Here's how the part is built. I have some questions about the finished solid (model axes, mm). A direction names the side the tool comes from. Give positions to 0.01 mm unless a question says otherwise; leave off trailing zeros. Loops run counter-clockwise (first coordinate to the right, second up) from the corner with the lowest first, then second, coordinate; pieces in that order, holes last.
Q1. Suppose I cut it at A-A (x = 51). List the corners of the cut face in (y, z) for me, and give its area (3 significant figures).
Q2. I'm going to push flat-ended pins straight in: P1, Ø19, axis at x = 57, z = -2, coming from the +Y side; P2, Ø8, axis at x = 30.5, y = -11.5, coming from the -Z side; P3, Ø8, axis at y = -11.5, z = -9, coming from the +X side. Where does each tip first touch, or does it pass through?
Q3. Suppose I cut it at C-C (x = 21). List the corners of the cut face in (y, z) for me.
Q4. I need wall thicknesses on probe 1 along Z at (x, y) = (51, -17); probe 2 along Z at (x, y) = (51, 12); probe 3 along Y at (x, z) = (49.5, 15). Which ranges of each line are inside material? Lowest first, please.
Q5. Thinking about a two-plate mould opening in Z: for faces 6 (the face through (20.354, 22.148, 8.24)), 7 (the face through (91, 19.5, 4)), 8 (the face through (48, -9.5, 32)), which applies, pulls with the +Z half, pulls with the -Z half, needs draft (parallel to the pull), parting line crosses it, or undercut?
Q6. Suppose I cut it at D-D (z = 15.5). List the corners of the cut face in (x, y) for me, and give its area (3 significant figures).
Q7. For faces 1 (the face through (18, 19.5, 0)), 2 (the face through (20.354, 22.148, -8.24)), 3 (the face through (23, 23, 0)), 4 (the face through (0, 0, 0)), 5 (the face through (6.2, 24.5, 10.1)), which set-ups out of +Z, -Z, +X, -X, +Y, -Y let a thin tool reach every point of the face, with its end or its side?
Q8. Suppose I cut it at B-B (y = 15). List the corners of the cut face in (x, z) for me.
Autodesk Inventor part; units mm, degrees
ref_plane "Work Plane2" through (0, -9.5, 0) normal (0, 1, 0) x (-1, 0, 0)
ref_plane "YZ Plane" through (0, 0, 0) normal (1, 0, 0) x (0, 1, 0)
ref_plane "XY Plane" through (0, 0, 0) normal (0, 0, 1) x (1, 0, 0)
sketch "Sketch2" plane through (0, 0, 0) normal (1, 0, 0) x (0, 1, 0)
  circle A0 centre (0, 0) radius 26.5
  dimension "d0" = 53
extrude "Extrusion1" add sketch "Sketch2" along normal blind 51
sketch "Sketch3" plane through (0, 0, 0) normal (0, 1, 0) x (-1, 0, 0)
  line L0 (-51, 26.5) -> (-51, -26.5)
  circle A0 centre (-51, 0) radius 48
  circle A1 centre (-51, 0) radius 39
  line L1 (-16.6387, 18.4473) -> (-22.6683, 1.8811)
  circle A2 centre (-17.5, 0) radius 5.5
  line L2 (0, 0) -> (-51, 0) construction
  line L3 (0, 26.5) -> (0, -26.5) construction
  line L4 (-16.6387, -18.4473) -> (-22.6683, -1.8811)
  circle A3 centre (-51, 0) radius 31.5
  point P0 (-22.6683, -1.8811)
  point P1 (-20.4946, 7.8532)
  point P2 (-20.4946, -7.8532)
  dimension "d4" = 78
  dimension "d7" = 11
  dimension "d3" = 96
  dimension "d8" = 17.5
  dimension "d9" = 140
  dimension "d15" = 63
ref_plane "Work Plane1" through (0, -26.5, 0) normal (0, 1, 0) x (-1, 0, 0)
extrude "Extrusion2" add sketch "Sketch3" along normal blind 46 from surface at -26.5 contours A0 | A2 A3 L1 A1 | A2 A3 | A1 L4 A3 A2 | L1 A3 L4 A1 | A3 A2 | A2 L1 A3 | A3 L4 A2 | L1 A2 L4 A3
ref_plane "Work Plane2" through (0, -9.5, 0) normal (0, 1, 0) x (-1, 0, 0)
extrude "Extrusion3" cut sketch "Sketch3" along normal up to surface (29 mm away) from surface at -9.5 contours A2 A3 L1 A1 | A2 A3 | A1 L4 A3 A2 | L1 A3 L4 A1 | A3 A2 | A2 L1 A3 | A3 L4 A2 | L1 A2 L4 A3
extrude "Extrusion4" cut sketch "Sketch3" along normal through all contours L1 A3 L4 A1 | L1 A2 L4 A3
extrude "Extrusion5" cut sketch "Sketch3" against normal blind 12 from surface at -9.5 contours A3 A2 | A2 L1 A3 | A3 L4 A2 | L1 A2 L4 A3 picked at (-20.6688, -0.7652)
properties part number "hip_right"
Solutions:
1. outline: (-26.5, -48) - (19.5, -48) - (19.5, -39) - (-9.5, -39) - (-9.5, -31.5) - (-21.5, -31.5) - (-21.5, 31.5) - (-9.5, 31.5) - (-9.5, 39) - (19.5, 39) - (19.5, 48) - (-26.5, 48) - close
1. area: 1,400 mm2
2. P1: stops at y = -21.5
2. P2: stops at z = -45.07
2. P3: stops at x = 98.74
3. outline: (-26.5, -37.47) - (19.5, -37.47) - (19.5, -24.92) - (-9.5, -24.92) - (-9.5, -9.6) - (-21.5, -9.6) - (-21.5, 9.6) - (-9.5, 9.6) - (-9.5, 24.92) - (19.5, 24.92) - (19.5, 37.47) - (-26.5, 37.47) - close; (19.5, -6.46) - (25.7, -6.46) arc R26.5 ccw to (25.7, 6.46) - (19.5, 6.46) - close
4. probe 1: z = -48 to -31.5, 31.5 to 48
4. probe 2: z = -48 to -39, 39 to 48
4. probe 3: y = -26.5 to -21.5
5. face 6: pulls with the +Z half
5. face 7: needs draft
5. face 8: undercut
6. outline: (0, -21.49) - (5.57, -21.49) - (5.57, -26.5) - (96.43, -26.5) - (96.43, 19.5) - (86.79, 19.5) - (86.79, -9.5) - (78.42, -9.5) - (78.42, -21.5) - (23.58, -21.5) - (23.58, -9.5) - (15.21, -9.5) - (15.21, 19.5) - (17.71, 19.5) - (17.71, 21.49) - (0, 21.49) - close
6. area: 1,710 mm2
7. face 1: none
7. face 2: -Z, +X, +Y
7. face 3: +X, +Y
7. face 4: +Z, -Z, -X, +Y, -Y
7. face 5: -X
8. outline: (0, -21.85) - (8.26, -21.85) arc R48 ccw (long way) to (8.26, 21.85) - (0, 21.85) - close; hole circle Ø78 at (51, 0)
